The listing builds one solid part. Answer for the finished solid, in the listing's coordinates (mm). A direction names the side the tool comes from. Give positions to 0.01 mm unless a question says otherwise; leave off trailing zeros. Write each loop counter-clockwise with the first axis right and the second up, starting at its lowest first coordinate (ties: lowest second). Pieces come first, ordered by that corner, then holes. Notation, with made-up numbers: (71.25, 40.5) -> (83.25, 40.5) arc R14 ccw to (83.25, 50.5) -> close; hole circle Ø10 at (1, 82.5). An arc over 180 degrees is marked (long way). Use CSV: the item, a comma, the result in double quotes. Start each with the question number.
from build123d import *

# Parameters (mm, degrees)
F1_DEPTH = 127
F2_W     = 43.000000447
F2_H     = 107.000000447
F3_ANGLE = 85


with BuildPart() as f1:
    # F0 (on Top) → F1 (new body)
    with BuildSketch(Plane.XY):
        with BuildLine():
            Line((58.2044105482, 24.109056239), (0, 0))
            Line((0, 0), (58.2044105482, -24.109056239))
            ThreePointArc((58.2044105482, -24.109056239), (63.0838940304, 0), (58.2044105482, 24.109056239))
        make_face()
    extrude(amount=F1_DEPTH)

    # F2 (on face) → F3 (revolve, cut)
    with BuildSketch(Plane(origin=(0, 0, 0), x_dir=(0.9238795325, -0.3826834324, 0), z_dir=(-0.3826834324, -0.9238795325, 0))):
        with Locations((31.5, 63.5)):
            Rectangle(F2_W, F2_H)
    revolve(axis=Axis((0, 0, 63.5), (0, 0, 1)), revolution_arc=F3_ANGLE, mode=Mode.SUBTRACT)


solid = f1.part
Q1. The mould has two halves that part along Z. Classify faces 3 (the face through (53, 0, 64)), 4 (the face through (3.641, 1.508, 62.611)), 5 (the face through (38, 0, 0)): +Z half, -Z half, draft (parallel to the pull), parting line (faces both ways), or undercut.
Q2. Section B-B on x = 20 is taken. Give the vertices of the cut face in (y, z), then the cut area to 3 significant figures.
Q3. Flat-ended cylindrical pins translate along their axes: pin 1 Ø1 at (x, z) = (51.5, 73) entering from -Y; pin 2 Ø8 at (y, z) = (-16.5, 101.5) entering from +X; pin 3 Ø1.5 at (x, z) = (55, 45.5) entering from +Y. Find the tip coordinate at first contact, or state that the pin passes through.
Q4. Section A-A on z = 49 is taken. Give the vertices of the cut face in (x, y).
Q5. For faces 1 (the face through (10, 0, 64)), 2 (the face through (2.826, -1.171, 62.611)), determine the directions among +Z, -Z, +X, -X, +Y, -Y from which every point of the face is accessible in a straight line to the end or side of a thin tool.
Q6. Section C-C on y = -2 is taken. Give the vertices of the cut face in (x, z).
Q7. Straight lines are drawn through the part: L1, parallel to Z at x = 41.5, y = 10.5; L2, parallel to X at y = -0.5, z = 22; L3, parallel to X at y = 4, z = 58. For each, find the intervals that lie inside material, in ascending order.
Q8. Section D-D on y = -17.5 is taken. Give the vertices of the cut face in (x, z).
Output:
1,face 3,"undercut"
1,face 4,"draft"
1,face 5,"-Z half"
2,outline,"(-8.28, 0) -> (8.28, 0) -> (8.28, 10) -> (-8.28, 10) -> close; (-8.28, 117) -> (8.28, 117) -> (8.28, 127) -> (-8.28, 127) -> close"
2,area,"331 mm²"
3,pin 1,"y = -21.54"
3,pin 2,"x = 61.81"
3,pin 3,"y = 23.09"
4,outline,"(0, 0) -> (9.24, -3.83) arc R10 ccw to (9.24, 3.83) -> close; (48.97, -20.28) -> (58.2, -24.11) arc R62 ccw to (58.2, 24.11) -> (48.97, 20.28) arc R53 cw to start"
5,face 1,"none"
5,face 2,"+Z, -Z, -X, -Y"
6,outline,"(4.83, 0) -> (63.05, 0) -> (63.05, 127) -> (4.83, 127) -> close; hole (9.8, 10) -> (52.96, 10) -> (52.96, 117) -> (9.8, 117) -> close"
7,L1,"0 to 10, 117 to 127"
7,L2,"1.21 to 9.99, 53 to 63.08"
7,L3,"52.85 to 62.95"
8,outline,"(42.25, 0) -> (60.56, 0) -> (60.56, 127) -> (42.25, 127) -> (42.25, 117) -> (50.03, 117) -> (50.03, 10) -> (42.25, 10) -> close"
